```python
from build123d import *

# Parameters (mm, degrees)
SKETCH1_W           = 20
SKETCH1_H           = 20
SKETCH1_W_2         = 17
SKETCH1_H_2         = 17
BOSS_EXTRUDE1_DEPTH = 40
SKETCH2_R           = 2.125
CUT_EXTRUDE1_DEPTH  = 46.82575695
SKETCH3_R           = 2.125
CUT_EXTRUDE2_DEPTH  = 46.82575695


with BuildPart() as part:
    # Sketch1 → Boss-Extrude1 (new body)
    with BuildSketch(Plane.XY):
        Rectangle(SKETCH1_W, SKETCH1_H)
        Rectangle(SKETCH1_W_2, SKETCH1_H_2, mode=Mode.SUBTRACT)
    extrude(amount=-BOSS_EXTRUDE1_DEPTH)

    # Sketch2 → Cut-Extrude1 (cut, through all)
    with BuildSketch(Plane(origin=(0, 10, 0), x_dir=(1, 0, 0), z_dir=(0, 1, 0))):
        with Locations(Location((0, 32, 0), (0, 0, 90))):
            Circle(SKETCH2_R)
        with Locations(Location((0, 16, 0), (0, 0, 270))):
            Circle(SKETCH2_R)
    extrude(amount=-CUT_EXTRUDE1_DEPTH, mode=Mode.SUBTRACT)

    # Sketch3 → Cut-Extrude2 (cut, through all)
    with BuildSketch(Plane(origin=(10, 0, 0), x_dir=(0, 0, -1), z_dir=(1, 0, 0))):
        with Locations((8, 0)):
            Circle(SKETCH3_R)
    extrude(amount=-CUT_EXTRUDE2_DEPTH, mode=Mode.SUBTRACT)


solid = part.part
```
Verification items for the finished model (mm, model axes). A direction names the side the tool comes from. Round coordinates to 2 decimals unless told otherwise and drop trailing zeros. Order: outer loops, then holes, each group sorted by start corner. A loop starts at its lowest first (then second) coordinate and runs counter-clockwise, first axis right, second up.
1) Cross-section at C-C, the plane y = 6.25. Record the cut outline in (x, z).
Geometry says:
outline: (-10, -40) - (-8.5, -40) - (-8.5, 0) - (-10, 0) - close; (8.5, -40) - (10, -40) - (10, 0) - (8.5, 0) - close
2) Depth check by flat-ended pin: pin 1 (3.5 mm diameter, centred on y = 0, z = -8, fed in from -X); pin 2 (12 mm diameter, centred on x = 0, z = -31, fed in from -Y). Enter the tip coordinate at first touch or a pass-through.
Geometry says:
pin 1: passes through
pin 2: stops at y = -10
3) Tool access check on faces 4 (the cylindrical face through (-0.638, 9.26, -34.027)), 5 (the flat face through (-8.5, 0, -20)). Record the directions out of +Z, -Z, +X, -X, +Y, -Y that give a thin tool (end or side, any length) a straight path to the whole face; none if there is none.
Geometry says:
face 4: +Y, -Y
face 5: +Z, -Z
4) Cross-section at B-B, the plane x = 0. Record the cut outline in (y, z) (3 decimals).
Geometry says:
outline: (-10, -40) - (-8.5, -40) - (-8.5, -34.125) - (-10, -34.125) - close; (-10, -29.875) - (-8.5, -29.875) - (-8.5, -18.125) - (-10, -18.125) - close; (-10, -13.875) - (-8.5, -13.875) - (-8.5, 0) - (-10, 0) - close; (8.5, -40) - (10, -40) - (10, -34.125) - (8.5, -34.125) - close; (8.5, -29.875) - (10, -29.875) - (10, -18.125) - (8.5, -18.125) - close; (8.5, -13.875) - (10, -13.875) - (10, 0) - (8.5, 0) - close
5) Cross-section at A-A, the plane z = -32. Record the cut outline in (x, y) (3 decimals), plus the area to 4 significant figures.
Geometry says:
outline: (-10, -10) - (-2.125, -10) - (-2.125, -8.5) - (-8.5, -8.5) - (-8.5, 8.5) - (-2.125, 8.5) - (-2.125, 10) - (-10, 10) - close; (2.125, -10) - (10, -10) - (10, 10) - (2.125, 10) - (2.125, 8.5) - (8.5, 8.5) - (8.5, -8.5) - (2.125, -8.5) - close
area: 98.25 mm2
6) Draft check along X on faces 1 (the flat face through (-10, 0, -20)), 2 (the flat face through (0, 8.5, -20)), 3 (the flat face through (0, 10, -20)). Enter one of: +X half, -X half, draft (parallel to the pull), parting line (faces both ways), or undercut.
Geometry says:
face 1: -X half
face 2: undercut
face 3: draft
7) Material ranges on line 1 (Y direction, x = -7.75, z = -33.5); line 2 (Y direction, x = 8.95, z = -8) (3 decimals), recorded low to high.
Geometry says:
line 1: y = -10 to -8.5, 8.5 to 10
line 2: y = -10 to -2.125, 2.125 to 10
8) Cross-section at D-D, the plane z = -26.5. Record the cut outline in (x, y).
Geometry says:
outline: (-10, -10) - (10, -10) - (10, 10) - (-10, 10) - close; hole (-8.5, -8.5) - (8.5, -8.5) - (8.5, 8.5) - (-8.5, 8.5) - close
